Part print with two shaded views. Sizes in mm from the minimum x, y, z corner. A direction names the side the tool comes from. Give positions to 0.01 mm unless a question says otherwise; leave off trailing zeros. Write each loop counter-clockwise with the first axis right and the second up, starting at its lowest first coordinate (ties: lowest second). Pieces come first, ordered by that corner, then holes. Notation, with made-up numbers: (-30, 2) -> (6, 2) arc R25 ccw to (6, 34) -> close; hole circle Ø10 at (-40, -10). An arc over 180 degrees is marked (long way). Write item = value, one per line. Start each with the question number.
Q1. Saw through at C-C, the plane y = 36.5. List the corners of the cut face in (x, z), then the cut area to 4 significant figures.
Q2. Drop flat-ended pins along their axis: P1, Ø10, axis at y = 33, z = 45.5, coming from the +X side; P2, Ø3, axis at x = 39.5, z = 46, coming from the +Y side. Give the stop position or say it passes through.
Q3. Saw through at B-B, the plane x = 45. List the corners of the cut face in (y, z), then the cut area to 3 significant figures.
Q4. Tool access for the marked faces 5 and 6: list every direction of +Z, -Z, +X, -X, +Y, -Y with a clear straight run to the whole face (end or side of a thin tool).
Q5. Saw through at D-D, the plane z = 75. List the corners of the cut face in (x, y) (1 decimal).
Q6. Mould opens along Z. For the marked faces 1, 2, 3 and 4 say: pulls with the +Z half, pulls with the -Z half, needs draft (parallel to the pull), parting line crosses it, or undercut.
Q7. Saw through at A-A, the plane z = 45. List the corners of the cut face in (x, y), then the cut area to 3 significant figures.
Q8. Wall check: line 1 (Z direction, x = 58, y = 21); line 2 (Y direction, x = 85, z = 44); line 3 (Z direction, x = 45, y = 41.7). Give the ranges that are in metal, low to high.
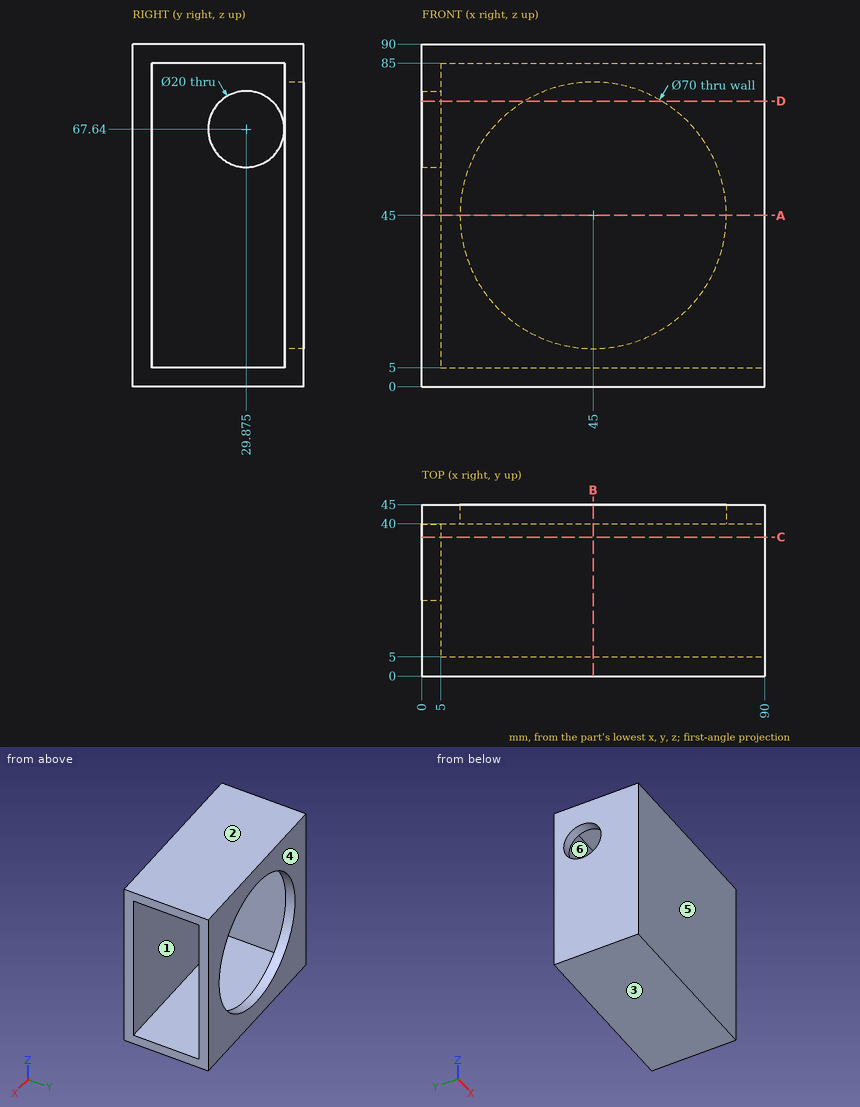
Report:
q1.outline = (0, 0) -> (90, 0) -> (90, 5) -> (5, 5) -> (5, 60.15) -> (0, 60.15) -> close; (0, 75.13) -> (5, 75.13) -> (5, 85) -> (90, 85) -> (90, 90) -> (0, 90) -> close
q1.area = 1,225 mm2
q2.P1 = 5
q2.P2 = 5
q3.outline = (0, 0) -> (45, 0) -> (45, 10) -> (40, 10) -> (40, 5) -> (5, 5) -> (5, 85) -> (40, 85) -> (40, 80) -> (45, 80) -> (45, 90) -> (0, 90) -> close
q3.area = 900 mm2
q4.face_5 = +Z, -Z, +X, -X, -Y
q4.face_6 = +X
q5.outline = (0, 0) -> (90, 0) -> (90, 5) -> (5, 5) -> (5, 23.1) -> (0, 23.1) -> close; (0, 36.6) -> (5, 36.6) -> (5, 40) -> (27, 40) -> (27, 45) -> (0, 45) -> close; (63, 40) -> (90, 40) -> (90, 45) -> (63, 45) -> close
q6.face_1 = undercut
q6.face_2 = pulls with the +Z half
q6.face_3 = pulls with the -Z half
q6.face_4 = needs draft
q7.outline = (0, 0) -> (90, 0) -> (90, 5) -> (5, 5) -> (5, 40) -> (10, 40) -> (10, 45) -> (0, 45) -> close; (80, 40) -> (90, 40) -> (90, 45) -> (80, 45) -> close
q7.area = 725 mm2
q8.line_1 = 0 to 5, 85 to 90
q8.line_2 = 0 to 5, 40 to 45
q8.line_3 = 0 to 10, 80 to 90
